```python
from build123d import *

# Parameters (mm, degrees)
SKETCH1_R           = 2.5527
BOSS_EXTRUDE1_DEPTH = 3.175
FILLET1_R           = 12.7


with BuildPart() as part:
    # Sketch1 → Boss-Extrude1 (new, symmetric)
    with BuildSketch(Plane(origin=(0, 0, 0), x_dir=(1, 0, 0), z_dir=(0, 1, 0))):
        with BuildLine():
            ThreePointArc((12.7, 12.7), (0, 0), (12.7, -12.7))
            Line((12.7, -12.7), (12.7, -38.1))
            ThreePointArc((12.7, -38.1), (25.4, -50.8), (38.1, -38.1))
            Line((38.1, -38.1), (38.1, -12.7))
            ThreePointArc((38.1, -12.7), (50.8, 0), (38.1, 12.7))
            Line((38.1, 12.7), (12.7, 12.7))
        make_face()
        with Locations(Location((25.4, -12.7, 0), (0, 0, 270))):
            Circle(SKETCH1_R, mode=Mode.SUBTRACT)
        with Locations(Location((12.7, 0, 0), (0, 0, 270))):
            Circle(SKETCH1_R, mode=Mode.SUBTRACT)
        with Locations(Location((38.1, 0, 0), (0, 0, 270))):
            Circle(SKETCH1_R, mode=Mode.SUBTRACT)
        with Locations(Location((25.4, 0, 0), (0, 0, 270))):
            Circle(SKETCH1_R, mode=Mode.SUBTRACT)
        with Locations(Location((25.4, -25.4, 0), (0, 0, 270))):
            Circle(SKETCH1_R, mode=Mode.SUBTRACT)
        with Locations(Location((25.4, -38.1, 0), (0, 0, 270))):
            Circle(SKETCH1_R, mode=Mode.SUBTRACT)
    extrude(amount=BOSS_EXTRUDE1_DEPTH, both=True)

    # Fillet1
    fillet1_edges = [part.edges().sort_by_distance(p)[0] for p in [
        (38.1, 0, 12.7),
        (12.7, 0, 12.7),
    ]]
    fillet(fillet1_edges, radius=FILLET1_R)


solid = part.part
```
For this review, take the finished solid that the model builds, in its own axes (mm). Give positions to 0.01 mm unless a question says otherwise; leave off trailing zeros. Write each loop counter-clockwise with the first axis right and the second up, starting at its lowest first coordinate (ties: lowest second). Pieces come first, ordered by that corner, then holes. Notation, with made-up numbers: M 83,4 L 87,4 A13 cw 87,12 Z; hole C 38,-2.75 d10. An arc over 180 degrees is marked long. Answer as CSV lines item,"result".
1. Consider section C-C, the plane z = 0. Write out the cut boundary in (x, y) (3 decimals).
Findings:
outline,"M 0,-3.175 L 10.147,-3.175 L 10.147,3.175 L 0,3.175 Z; M 15.253,-3.175 L 22.847,-3.175 L 22.847,3.175 L 15.253,3.175 Z; M 27.953,-3.175 L 35.547,-3.175 L 35.547,3.175 L 27.953,3.175 Z; M 40.653,-3.175 L 50.8,-3.175 L 50.8,3.175 L 40.653,3.175 Z"
2. Consider section B-B, the plane x = 25.4. Write out the cut boundary in (y, z) (3 decimals), then the cut area to 3 significant figures.
Findings:
outline,"M -3.175,-12.7 L 3.175,-12.7 L 3.175,-2.553 L -3.175,-2.553 Z; M -3.175,2.553 L 3.175,2.553 L 3.175,10.147 L -3.175,10.147 Z; M -3.175,15.253 L 3.175,15.253 L 3.175,22.847 L -3.175,22.847 Z; M -3.175,27.953 L 3.175,27.953 L 3.175,35.547 L -3.175,35.547 Z; M -3.175,40.653 L 3.175,40.653 L 3.175,50.8 L -3.175,50.8 Z"
area,"274 mm2"
3. Wall thickness on line 1 (X direction, y = 2, z = 0); line 2 (X direction, y = -1.5, z = 12.7); line 3 (X direction, y = 2.75, z = 22): over which ranges is each line inside the solid? List them lowest first.
Findings:
line 1,"x = 0 to 10.15, 15.25 to 22.85, 27.95 to 35.55, 40.65 to 50.8"
line 2,"x = 8.65 to 22.85, 27.95 to 42.15"
line 3,"x = 12.7 to 38.1"
4. Consider section D-D, the plane y = -2. Write out the cut boundary in (x, z).
Findings:
outline,"M 6.35,11 A12.7 ccw 12.7,-12.7 L 38.1,-12.7 A12.7 ccw 44.45,11 A12.7 cw 38.1,22 L 38.1,38.1 A12.7 ccw 12.7,38.1 L 12.7,22 A12.7 cw Z; hole C 12.7,0 d5.11; hole C 25.4,0 d5.11; hole C 25.4,12.7 d5.11; hole C 25.4,25.4 d5.11; hole C 25.4,38.1 d5.11; hole C 38.1,0 d5.11"
5. For pin 1 (3 mm diameter, centred on x = 25.4, z = 12.7, fed in from +Y); pin 2 (1.5 mm diameter, centred on y = -2, z = -5.5, fed in from -X); pin 3 (1.9 mm diameter, centred on y = -1, z = 32, fed in from -X); pin 4 (1.5 mm diameter, centred on x = 40.5, y = 2.5, fed in from +Z), all flat-tipped, find the tip position at first contact; note any pin that passes through.
Findings:
pin 1,"passes through"
pin 2,"stops at x = 0.92"
pin 3,"stops at x = 12.7"
pin 4,"stops at z = 15.74"
6. Consider section A-A, the plane z = 25.4. Write out the cut boundary in (x, y) (3 decimals).
Findings:
outline,"M 12.7,-3.175 L 22.847,-3.175 L 22.847,3.175 L 12.7,3.175 Z; M 27.953,-3.175 L 38.1,-3.175 L 38.1,3.175 L 27.953,3.175 Z"
7. Draft analysis for pull direction X (two halves, no side actions). For faces 1 (the cylindrical face through (27.93, -0.04, -0.33)), 2 (the flat face through (12.7, 0, 30)), 3 (the flat face through (38.1, 0, 30)), 4 (the flat face through (26, 0, -12.7)), state which applies: +X half, -X half, draft (parallel to the pull), parting line (faces both ways), or undercut.
Findings:
face 1,"undercut"
face 2,"-X half"
face 3,"+X half"
face 4,"draft"
